```python
from build123d import *

# Parameters (mm, degrees)
EXTRUDE_1_DEPTH       = 400
HOLE_WIZARD_10_32_1_D = 4.0386


with BuildPart() as part:
    # 草圖1 → 填料-伸長1 (new body)
    with BuildSketch(Plane(origin=(0, 0, 0), x_dir=(1, 0, 0), z_dir=(0, 1, 0))):
        with BuildLine():
            Line((8.5, 9), (-8.5, 9))
            ThreePointArc((-8.5, 9), (-17.5, 0), (-8.5, -9))
            Line((-8.5, -9), (8.5, -9))
            ThreePointArc((8.5, -9), (17.5, 0), (8.5, 9))
        make_face()
        with BuildLine():
            Line((8.5, -7.4), (-8.5, -7.4))
            ThreePointArc((-8.5, -7.4), (-15.9, 0), (-8.5, 7.4))
            Line((-8.5, 7.4), (8.5, 7.4))
            ThreePointArc((8.5, 7.4), (15.9, 0), (8.5, -7.4))
        make_face(mode=Mode.SUBTRACT)
    extrude(amount=EXTRUDE_1_DEPTH)

    # #10-32 螺紋孔1 (through all)
    with Locations(Plane.XY.offset(9)):
        with Locations((0, 30), (0, 15), (0, 385), (0, 370)):
            Hole(HOLE_WIZARD_10_32_1_D / 2)


solid = part.part
```
Geometry: final body of the model. Coordinates: model frame, mm. A direction names the side the tool comes from. Coordinates: 2 decimals unless noted, no trailing zeros. Order: outer loops, then holes, each group sorted by start corner. A loop starts at its lowest first (then second) coordinate and runs counter-clockwise, first axis right, second up. Notation, with made-up numbers: (50, 69.25) -> (63, 69.25) arc R29 ccw to (63, 108.25) -> close; hole circle Ø5 at (64, -21). An arc over 180 degrees is marked (long way). Write each question's results on one line, items separated by ' | '. Start each with the question number.
1) Set-up query: faces 1 (the cylindrical face through (-15.9, 197.2, 0.16)), 2 (the flat face through (0, 197, -9)). Return all of +Z, -Z, +X, -X, +Y, -Y with unobstructed straight access to the full face (end or side cutting, diameter ignored); none if empty.
2) Mould query, pull axis Z, two halves, no side actions, for faces 3 (the flat face through (0, 400, 8)), 4 (the cylindrical face through (-17.498, 197.2, -0.198)), 5 (the flat face through (0, 197, -7.4)). Classes: released by +Z, released by -Z, zero draft, split by the parting line, or undercut.
3) Cut plane A-A, the plane y = 226. Output: boundary loops of the cut face in (x, z), and give its area (3 significant figures).
4) Cut plane B-B, the plane z = 0. Output: boundary loops of the cut face in (x, y).
5) Material intervals for line 1 along Y through (x, z) = (0, 8.2); line 2 along X through (y, z) = (372, -0.5); line 3 along Z through (x, y) = (-1, 251), sorted ascending.
6) First-contact query: pin 1 (4.5 mm diameter, centred on x = 0, y = 370, fed in from -Z); pin 2 (3 mm diameter, centred on y = 148.5, z = 5, fed in from -X); pin 3 (1 mm diameter, centred on x = 13, y = 52, fed in from -Z). Flat tips, straight axial feed; report the tip coordinate or a pass-through.
Checks:
1) face 1: +Y, -Y | face 2: -Z, +X, -X, +Y, -Y
2) face 3: zero draft | face 4: split by the parting line | face 5: undercut
3) outline: (-8.5, -9) -> (8.5, -9) arc R9 ccw to (8.5, 9) -> (-8.5, 9) arc R9 ccw to start; hole (-8.5, -7.4) -> (8.5, -7.4) arc R7.4 ccw to (8.5, 7.4) -> (-8.5, 7.4) arc R7.4 ccw to start | area: 137 mm^2
4) outline: (-17.5, 0) -> (-15.9, 0) -> (-15.9, 400) -> (-17.5, 400) -> close; (15.9, 0) -> (17.5, 0) -> (17.5, 400) -> (15.9, 400) -> close
5) line 1: 0 to 12.98, 17.02 to 27.98, 32.02 to 367.98, 372.02 to 382.98, 387.02 to 400 | line 2: -17.49 to -15.88, 15.88 to 17.49 | line 3: -9 to -7.4, 7.4 to 9
6) pin 1: z = -9 | pin 2: x = -16.79 | pin 3: z = -8.06
